```python
from build123d import *

# Parameters (mm, degrees)
SKETCH1_R           = 24
EXTRUDE1_DEPTH      = 5
SKETCH2_R           = 24
EXTRUDE2_DEPTH      = 8
SKETCH3_R           = 2.5
SKETCH3_R_2         = 3.7
EXTRUDE3_DEPTH      = 7
SKETCH5_R           = 3
EXTRUDE6_DEPTH      = 10
SKETCH6_R           = 3.175
EXTRUDE7_DEPTH      = 3
SKETCH7_R           = 1.7
EXTRUDE8_DEPTH      = 8
EXTRUDE8_DEPTH_BACK = 3
SKETCH8_W           = 3.4
SKETCH8_H           = 3
EXTRUDE9_DEPTH      = 3
EXTRUDE10_DEPTH     = 1


with BuildPart() as part:
    # Sketch1 → Extrude1 (new body)
    with BuildSketch(Plane.XY):
        Circle(SKETCH1_R)
    extrude(amount=EXTRUDE1_DEPTH)

    # Sketch2 → Extrude2 (add)
    with BuildSketch(Plane.XY.offset(5)):
        Circle(SKETCH2_R)
        with BuildLine():
            Line((-2.5, 0), (-10.5, 0))
            Line((-10.5, 0), (-10.5, -5))
            Line((-10.5, -5), (10.5, -5))
            Line((10.5, -5), (10.5, 0))
            Line((10.5, 0), (2.5, 0))
            ThreePointArc((2.5, 0), (0, -2.5), (-2.5, 0))
        make_face(mode=Mode.SUBTRACT)
    extrude(amount=EXTRUDE2_DEPTH)

    # Sketch3 → Extrude3 (add)
    with BuildSketch(Plane.XY.offset(13)):
        Circle(SKETCH3_R)
        with Locations((-7.9375, 7.9375)):
            Circle(SKETCH3_R_2)
        with Locations((7.9375, 7.9375)):
            Circle(SKETCH3_R_2)
        with Locations((0, -11.1125)):
            Circle(SKETCH3_R_2)
    extrude(amount=EXTRUDE3_DEPTH)

    # Sketch5 → Extrude6 (add)
    with BuildSketch(Plane.XY.offset(20)):
        with Locations((-7.9375, 7.9375)):
            Circle(SKETCH5_R)
        with Locations((7.9375, 7.9375)):
            Circle(SKETCH5_R)
        with Locations((0, -11.1125)):
            Circle(SKETCH5_R)
    extrude(amount=EXTRUDE6_DEPTH)

    # Sketch6 → Extrude7 (cut)
    with BuildSketch(Plane(origin=(0, 0, 0), x_dir=(-1, 0, 0), z_dir=(0, 0, -1))):
        with Locations((0, 12.7)):
            Circle(SKETCH6_R)
        with Locations((7.9375, -11.1125)):
            Circle(SKETCH6_R)
        with Locations((-7.9375, -11.1125)):
            Circle(SKETCH6_R)
    extrude(amount=-EXTRUDE7_DEPTH, mode=Mode.SUBTRACT)

    # Sketch7 → Extrude8 (cut, two sides)
    with BuildSketch(Plane.XZ) as extrude8_sk:
        with Locations((-6.5, 9)):
            Circle(SKETCH7_R)
        with Locations((6.5, 9)):
            Circle(SKETCH7_R)
    extrude(amount=EXTRUDE8_DEPTH, mode=Mode.SUBTRACT)
    extrude(extrude8_sk.sketch, amount=-EXTRUDE8_DEPTH_BACK, mode=Mode.SUBTRACT)

    # Sketch8 → Extrude9 (cut)
    with BuildSketch(Plane.XY.offset(13)):
        with Locations((-6.5, -6.5)):
            Rectangle(SKETCH8_W, SKETCH8_H)
        with Locations((6.5, -6.5)):
            Rectangle(SKETCH8_W, SKETCH8_H)
    extrude(amount=-EXTRUDE9_DEPTH, mode=Mode.SUBTRACT)

    # Sketch9 → Extrude10 (cut)
    with BuildSketch(Plane.XY.offset(13)):
        Polygon((24, 0), (24, -1.5), (15.5, -1.5), (15.5, 1.5), (24, 1.5), align=None)
        Polygon((22.17310878, 9.184402377), (22.747133929, 7.798583078), (14.894157902, 4.545773903), (13.746107605, 7.3174125), (21.599083632, 10.570221676), align=None)
        Polygon((16.970562748, 16.970562748), (18.03122292, 15.909902577), (12.02081528, 9.899494937), (9.899494937, 12.02081528), (15.909902577, 18.03122292), align=None)
        Polygon((9.184402377, 22.17310878), (10.570221676, 21.599083632), (7.3174125, 13.746107605), (4.545773903, 14.894157902), (7.798583078, 22.747133929), align=None)
        Polygon((0, 24), (1.5, 24), (1.5, 15.5), (-1.5, 15.5), (-1.5, 24), align=None)
        Polygon((-9.184402377, 22.17310878), (-7.798583078, 22.747133929), (-4.545773903, 14.894157902), (-7.3174125, 13.746107605), (-10.570221676, 21.599083632), align=None)
        Polygon((-16.970562748, 16.970562748), (-15.909902577, 18.03122292), (-9.899494937, 12.02081528), (-12.02081528, 9.899494937), (-18.03122292, 15.909902577), align=None)
        Polygon((-22.17310878, 9.184402377), (-21.599083632, 10.570221676), (-13.746107605, 7.3174125), (-14.894157902, 4.545773903), (-22.747133929, 7.798583078), align=None)
        Polygon((-24, 0), (-24, 1.5), (-15.5, 1.5), (-15.5, -1.5), (-24, -1.5), align=None)
        Polygon((-22.17310878, -9.184402377), (-22.747133929, -7.798583078), (-14.894157902, -4.545773903), (-13.746107605, -7.3174125), (-21.599083632, -10.570221676), align=None)
        Polygon((-16.970562748, -16.970562748), (-15.909902577, -18.03122292), (-9.899494937, -12.02081528), (-12.02081528, -9.899494937), (-18.03122292, -15.909902577), align=None)
        Polygon((-9.184402377, -22.17310878), (-7.798583078, -22.747133929), (-4.545773903, -14.894157902), (-7.3174125, -13.746107605), (-10.570221676, -21.599083632), align=None)
        Polygon((0, -24), (1.5, -24), (1.5, -15.5), (-1.5, -15.5), (-1.5, -24), align=None)
        Polygon((9.184402377, -22.17310878), (10.570221676, -21.599083632), (7.3174125, -13.746107605), (4.545773903, -14.894157902), (7.798583078, -22.747133929), align=None)
        Polygon((16.970562748, -16.970562748), (18.03122292, -15.909902577), (12.02081528, -9.899494937), (9.899494937, -12.02081528), (15.909902577, -18.03122292), align=None)
        Polygon((22.17310878, -9.184402377), (22.747133929, -7.798583078), (14.894157902, -4.545773903), (13.746107605, -7.3174125), (21.599083632, -10.570221676), align=None)
    extrude(amount=-EXTRUDE10_DEPTH, mode=Mode.SUBTRACT)


solid = part.part
```
CAD build for the part. Positions are in the model's coordinates, mm. A direction names the side the tool comes from. Round coordinates to 2 decimals unless told otherwise and drop trailing zeros. Order: outer loops, then holes, each group sorted by start corner. A loop starts at its lowest first (then second) coordinate and runs counter-clockwise, first axis right, second up. Notation, with made-up numbers: (49.5, 85) - (66.5, 85) arc R31 ccw to (66.5, 115) - close; hole circle Ø5 at (88.5, 83.5). An arc over 180 degrees is marked (long way). Answer in a Markdown table with one row per item. Add a question column.
(1) Band-saw the part on D-D on z = 24.5. List the corners of the cut face in (x, y).
(2) Probe L1, parallel to Y at x = 0, z = 0.7 (3 decimals); L2, parallel to Z at x = 6.5, y = 0.65; L3, parallel to X at y = -6.9, z = 9. List the from-to ranges inside material, lowest first. Write a range as [from, to].
(3) Band-saw the part on A-A on z = 9. List the corners of the cut face in (x, y), and give its area (3 significant figures).
(4) Band-saw the part on B-B on x = 0. List the corners of the cut face in (y, z) (1 decimal).
(5) 3-axis set-ups, long thin cutter, end or side, ignore diameter. For faces 5 (the face through (10.5, -3, 9)), 6 (the face through (-20, 0, 12)), 7 (the face through (-7, 3, 9)), 8 (the face through (-1.5, 9.9, 1.5)): which of +Z, -Z, +X, -X, +Y, -Y reach the whole face in a straight line?
(6) Drop flat-ended pins along their axis: pin 1 Ø12 at (x, z) = (15, 26.5) entering from -Y; pin 2 Ø6.5 at (x, y) = (-8, 16.5) entering from +Z; pin 3 Ø1 at (y, z) = (11, 25.5) entering from -X; pin 4 Ø8 at (y, z) = (-2.5, 6.5) entering from -X. Give the stop position or say it passes through.
(7) Mould opens along X. For faces 1 (the face through (-5.076, 8.839, 24.93)), 2 (the face through (15.05, -12.93, 12.51)), 3 (the face through (0, 0, 0)), 4 (the face through (22.17, -9.19, 6.41)) say: +X half, -X half, draft (parallel to the pull), parting line (faces both ways), or undercut.
(8) Band-saw the part on C-C on y = 12.7. List the corners of the cut face in (x, z) (3 decimals), and give its area (3 significant figures).
Data:
| question | item | result |
|---|---|---|
| 1 | outline | circle Ø6 at (-7.94, 7.94); circle Ø6 at (0, -11.11); circle Ø6 at (7.94, 7.94) |
| 2 | L1 | y = [-24, 9.525], [15.875, 24] |
| 2 | L2 | z = [0, 7.3], [10.7, 13] |
| 2 | L3 | x = [-22.99, -8.2], [-4.8, 4.8], [8.2, 22.99] |
| 3 | outline | circle Ø48 at (0, 0); hole (-10.5, -5) - (-8.2, -5) - (-8.2, -8) - (-4.8, -8) - (-4.8, -5) - (4.8, -5) - (4.8, -8) - (8.2, -8) - (8.2, -5) - (10.5, -5) - (10.5, 0) - (8.2, 0) - (8.2, 3) - (4.8, 3) - (4.8, 0) - (2.5, 0) arc R2.5 cw to (-2.5, 0) - (-4.8, 0) - (-4.8, 3) - (-8.2, 3) - (-8.2, 0) - (-10.5, 0) - close |
| 3 | area | 1,670 mm^2 |
| 4 | outline | (-24, 0) - (9.5, 0) - (9.5, 3) - (15.9, 3) - (15.9, 0) - (24, 0) - (24, 12) - (15.5, 12) - (15.5, 13) - (2.5, 13) - (2.5, 20) - (-2.5, 20) - (-2.5, 5) - (-5, 5) - (-5, 13) - (-7.4, 13) - (-7.4, 20) - (-8.1, 20) - (-8.1, 30) - (-14.1, 30) - (-14.1, 20) - (-14.8, 20) - (-14.8, 13) - (-15.5, 13) - (-15.5, 12) - (-24, 12) - close |
| 5 | face 5 | +Z |
| 5 | face 6 | +Z, -X |
| 5 | face 7 | none |
| 5 | face 8 | -Z |
| 6 | pin 1 | stops at y = 5.13 |
| 6 | pin 2 | stops at z = 13 |
| 6 | pin 3 | stops at x = -9.5 |
| 6 | pin 4 | stops at x = -24 |
| 7 | face 1 | undercut |
| 7 | face 2 | undercut |
| 7 | face 3 | draft |
| 7 | face 4 | parting line |
| 8 | outline | (-20.364, 0) - (-3.175, 0) - (-3.175, 3) - (3.175, 3) - (3.175, 0) - (20.364, 0) - (20.364, 13) - (14.821, 13) - (14.821, 12) - (10.579, 12) - (10.579, 13) - (-10.579, 13) - (-10.579, 12) - (-14.821, 12) - (-14.821, 13) - (-20.364, 13) - close |
| 8 | area | 502 mm^2 |
